Here's how the part is built. I have some questions about the finished solid (model axes, mm). Face numbers are marked on the shaded views. A direction names the side the tool comes from. Round coordinates to 2 decimals unless told otherwise and drop trailing zeros. Loops run counter-clockwise (first coordinate to the right, second up) from the corner with the lowest first, then second, coordinate; pieces in that order, holes last. Notation, with made-up numbers: (18, 81.5) - (61, 81.5) arc R17 cw to (61, 96.5) - close; hole circle Ø1 at (-31, 63). An arc over 180 degrees is marked (long way). Return JSON: item names as keys, results as strings. Group by question number.
```python
from build123d import *

# Parameters (mm, degrees)
SKETCH1_R      = 2.5
SKETCH1_R_2    = 6.85
EXTRUDE1_DEPTH = 100


with BuildPart() as part:
    # Sketch1 → Extrude1 (new body)
    with BuildSketch(Plane.XY):
        Polygon((-20, -24), (-16, -24), (-16, -31), (-13.828427, -31), (-10, -27.171573), (-10, -12.828427), (-13.828427, -9), (-16, -9), (-16, -16), (-20, -16), (-20, 16), (-16, 16), (-16, 9), (-13.828427, 9), (-10, 12.828427), (-10, 27.171573), (-13.828427, 31), (-16, 31), (-16, 24), (-20, 24), (-20, 40), (-4, 40), (-4, 36), (-11, 36), (-11, 33.828427), (-7.171573, 30), (7.171573, 30), (11, 33.828427), (11, 36), (4, 36), (4, 40), (20, 40), (20, 24), (16, 24), (16, 31), (13.828427, 31), (10, 27.171573), (10, 12.828427), (13.828427, 9), (16, 9), (16, 16), (20, 16), (20, -16), (16, -16), (16, -9), (13.828427, -9), (10, -12.828427), (10, -27.171573), (13.828427, -31), (16, -31), (16, -24), (20, -24), (20, -40), (4, -40), (4, -36), (11, -36), (11, -33.828427), (7.171573, -30), (-7.171573, -30), (-11, -33.828427), (-11, -36), (-4, -36), (-4, -40), (-20, -40), align=None)
        with Locations((-15.5, -35.5)):
            Circle(SKETCH1_R, mode=Mode.SUBTRACT)
        with Locations((-15.5, 35.5)):
            Circle(SKETCH1_R, mode=Mode.SUBTRACT)
        with Locations((15.5, -35.5)):
            Circle(SKETCH1_R, mode=Mode.SUBTRACT)
        with Locations((15.5, 35.5)):
            Circle(SKETCH1_R, mode=Mode.SUBTRACT)
        with Locations((0, -20)):
            Circle(SKETCH1_R_2, mode=Mode.SUBTRACT)
        with Locations((0, 20)):
            Circle(SKETCH1_R_2, mode=Mode.SUBTRACT)
        Polygon((-8.87868, -9), (8.87868, -9), (12.37868, -5.5), (16, -5.5), (16, 5.5), (12.37868, 5.5), (8.87868, 9), (-8.87868, 9), (-12.37868, 5.5), (-16, 5.5), (-16, -5.5), (-12.37868, -5.5), align=None, mode=Mode.SUBTRACT)
    extrude(amount=-EXTRUDE1_DEPTH)


solid = part.part
```
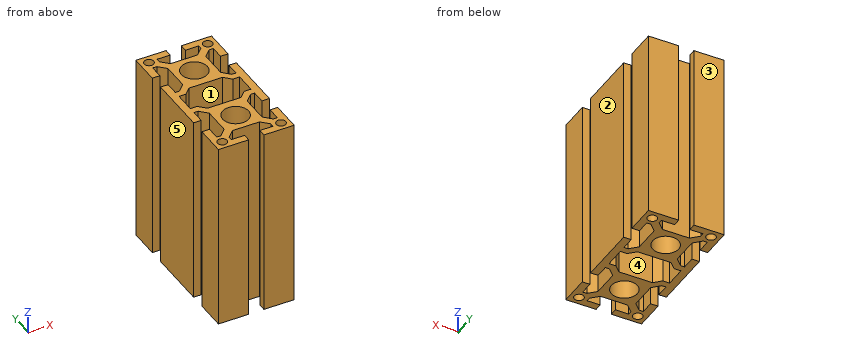
Q1. Will this pin go through, and if not, where does the flat tip stop? pin 1 Ø4 at (x, y) = (-15.5, -35.5) entering from -Z.
Q2. Imagine slicing it at D-D, the plane y = -18.5. List the corners of the cut face in (x, z) for me, and give its area (3 significant figures).
Q3. For the marked faces 4 and 5, which set-ups out of +Z, -Z, +X, -X, +Y, -Y let a thin tool reach every point of the face, with its end or its side?
Q4. Imagine slicing it at C-C, the plane z = -45.5. Give the number of separate pieces and of enclosed holes in the cut face, and give its area (3 significant figures).
Q5. If we mould it in two halves opening along X, with no side actions, what happens to the marked faces 1, 2 and 3? For each: +X half, -X half, draft (parallel to the pull), parting line (faces both ways), or undercut.
Q6. Please list where these lines run through material, in increasing order: line 1 (X direction, y = -10, z = -96); line 2 (X direction, y = -10.5, z = -4); line 3 (Y direction, x = -13.5, z = -35).
Q7. Imagine slicing it at A-A, the plane y = 20. List the corners of the cut face in (x, z) for me.
Q8. Imagine slicing it at B-B, the plane x = 2. List the corners of the cut face in (y, z) for me, and give its area (3 significant figures).
Output values:
{
 "1": {"pin 1": "passes through"},
 "2": {"outline": "(-10, -100) - (-6.68, -100) - (-6.68, 0) - (-10, 0) - close; (6.68, -100) - (10, -100) - (10, 0) - (6.68, 0) - close", "area": "663 mm^2"},
 "3": {"face 4": "+Z, -Z", "face 5": "+Z, -Z, -X, +Y, -Y"},
 "4": {"separate pieces": "1", "enclosed holes": "7", "area": "1,430 mm^2"},
 "5": {"face 1": "undercut", "face 2": "+X half", "face 3": "draft"},
 "6": {"line 1": "x = -20 to -16, -12.83 to 12.83, 16 to 20", "line 2": "x = -20 to -16, -12.33 to 12.33, 16 to 20", "line 3": "y = -40 to -37, -34 to -30.67, -9.33 to -5.5, 5.5 to 9.33, 30.67 to 34, 37 to 40"},
 "7": {"outline": "(-10, -100) - (-6.85, -100) - (-6.85, 0) - (-10, 0) - close; (6.85, -100) - (10, -100) - (10, 0) - (6.85, 0) - close"},
 "8": {"outline": "(-30, -100) - (-26.55, -100) - (-26.55, 0) - (-30, 0) - close; (-13.45, -100) - (-9, -100) - (-9, 0) - (-13.45, 0) - close; (9, -100) - (13.45, -100) - (13.45, 0) - (9, 0) - close; (26.55, -100) - (30, -100) - (30, 0) - (26.55, 0) - close", "area": "1,580 mm^2"}
}
